```python
from build123d import *

# Parameters (mm, degrees)
F1_W     = 5.5
F1_H     = 15
F1_R     = 1.45
F2_DEPTH = 4
F3_DEPTH = 14
F4_R     = 2.5
F5_R     = 5
F6_W     = 42.5
F6_H     = 2
F7_DEPTH = 4
F8_SIZE2 = 4
F8_SIZE  = 20
F9_R     = 1


with BuildPart() as f2:
    # F1 (on Top) → F2 (new body)
    with BuildSketch(Plane.XY):
        with BuildLine():
            ThreePointArc((-44, 27), (-42.232233047, 26.267766953), (-41.5, 24.5))
            ThreePointArc((-41.5, 24.5), (-44, 22), (-46.5, 24.5))
            Line((-46.5, 24.5), (-46.5, -24.5))
            ThreePointArc((-46.5, -24.5), (-44, -22), (-41.5, -24.5))
            ThreePointArc((-41.5, -24.5), (-42.232233047, -26.267766953), (-44, -27))
            Line((-44, -27), (14, -27))
            Line((14, -27), (16.5, -27))
            Line((16.5, -27), (57.5, -27))
            Line((57.5, -27), (57.5, 27))
            Line((57.5, 27), (16.5, 27))
            Line((16.5, 27), (14, 27))
            Line((14, 27), (-44, 27))
        make_face()
        with BuildLine():
            ThreePointArc((16.5, -24.5), (15.767766953, -26.267766953), (14, -27))
            ThreePointArc((14, -27), (12.232233047, -22.732233047), (16.5, -24.5))
        make_face(mode=Mode.SUBTRACT)
        with Locations((47.5, -12)):
            Rectangle(F1_W, F1_H, mode=Mode.SUBTRACT)
        Polygon((11.5, -19.400605268), (11.5, -22), (8.368910891, -22), (-38.368910891, -22), (-41.5, -22), (-41.5, -19.400605268), (-41.5, 19.400605268), (-41.5, 22), (-38.368910891, 22), (8.368910891, 22), (11.5, 22), (11.5, 19.400605268), align=None, mode=Mode.SUBTRACT)
        with Locations((47.5, 12)):
            Rectangle(F1_W, F1_H, mode=Mode.SUBTRACT)
        with BuildLine():
            ThreePointArc((16.5, 24.5), (12.232233047, 22.732233047), (14, 27))
            ThreePointArc((14, 27), (15.767766953, 26.267766953), (16.5, 24.5))
        make_face(mode=Mode.SUBTRACT)
        Polygon((-41.5, 19.400605268), (-18.131089109, 0), (-15, 2.599394732), (-38.368910891, 22), (-41.5, 22), align=None)
        Polygon((-11.868910891, 0), (11.5, 19.400605268), (11.5, 22), (8.368910891, 22), (-15, 2.599394732), align=None)
        Polygon((8.368910891, -22), (11.5, -22), (11.5, -19.400605268), (-11.868910891, 0), (-15, -2.599394732), align=None)
        Polygon((-41.5, -22), (-38.368910891, -22), (-15, -2.599394732), (-18.131089109, 0), (-41.5, -19.400605268), align=None)
        with BuildLine():
            ThreePointArc((16.5, 24.5), (15.767766953, 26.267766953), (14, 27))
            ThreePointArc((14, 27), (12.232233047, 22.732233047), (16.5, 24.5))
        make_face()
        with Locations((14, 24.5)):
            Circle(F1_R, mode=Mode.SUBTRACT)
        with BuildLine():
            ThreePointArc((16.5, -24.5), (12.232233047, -22.732233047), (14, -27))
            ThreePointArc((14, -27), (15.767766953, -26.267766953), (16.5, -24.5))
        make_face()
        with Locations((14, -24.5)):
            Circle(F1_R, mode=Mode.SUBTRACT)
        with BuildLine():
            ThreePointArc((-46.5, 24.5), (-44, 22), (-41.5, 24.5))
            ThreePointArc((-41.5, 24.5), (-42.232233047, 26.267766953), (-44, 27))
            ThreePointArc((-44, 27), (-45.767766953, 26.267766953), (-46.5, 24.5))
        make_face()
        with Locations((-44, 24.5)):
            Circle(F1_R, mode=Mode.SUBTRACT)
        with BuildLine():
            ThreePointArc((-41.5, -24.5), (-44, -22), (-46.5, -24.5))
            ThreePointArc((-46.5, -24.5), (-45.767766953, -26.267766953), (-44, -27))
            ThreePointArc((-44, -27), (-42.232233047, -26.267766953), (-41.5, -24.5))
        make_face()
        with Locations((-44, -24.5)):
            Circle(F1_R, mode=Mode.SUBTRACT)
        Polygon((-18.131089109, 0), (-15, -2.599394732), (-11.868910891, 0), (-15, 2.599394732), align=None)
    extrude(amount=F2_DEPTH)

    # F1 (on Top) → F3 (join)
    with BuildSketch(Plane.XY):
        with BuildLine():
            ThreePointArc((-46.5, 24.5), (-44, 22), (-41.5, 24.5))
            ThreePointArc((-41.5, 24.5), (-42.232233047, 26.267766953), (-44, 27))
            ThreePointArc((-44, 27), (-45.767766953, 26.267766953), (-46.5, 24.5))
        make_face()
        with Locations((-44, 24.5)):
            Circle(F1_R, mode=Mode.SUBTRACT)
        with BuildLine():
            ThreePointArc((16.5, 24.5), (15.767766953, 26.267766953), (14, 27))
            ThreePointArc((14, 27), (12.232233047, 22.732233047), (16.5, 24.5))
        make_face()
        with Locations((14, 24.5)):
            Circle(F1_R, mode=Mode.SUBTRACT)
        with BuildLine():
            ThreePointArc((16.5, -24.5), (12.232233047, -22.732233047), (14, -27))
            ThreePointArc((14, -27), (15.767766953, -26.267766953), (16.5, -24.5))
        make_face()
        with Locations((14, -24.5)):
            Circle(F1_R, mode=Mode.SUBTRACT)
        with BuildLine():
            ThreePointArc((-41.5, -24.5), (-44, -22), (-46.5, -24.5))
            ThreePointArc((-46.5, -24.5), (-45.767766953, -26.267766953), (-44, -27))
            ThreePointArc((-44, -27), (-42.232233047, -26.267766953), (-41.5, -24.5))
        make_face()
        with Locations((-44, -24.5)):
            Circle(F1_R, mode=Mode.SUBTRACT)
    extrude(amount=F3_DEPTH)

    # F4
    f4_edges = [f2.edges().sort_by_distance(p)[0] for p in [
        (44.75, 19.5, 2),
        (50.25, 19.5, 2),
        (50.25, 4.5, 2),
        (44.75, 4.5, 2),
        (44.75, -19.5, 2),
        (50.25, -19.5, 2),
        (50.25, -4.5, 2),
        (44.75, -4.5, 2),
    ]]
    fillet(f4_edges, radius=F4_R)

    # F5
    f5_edges = [f2.edges().sort_by_distance(p)[0] for p in [
        (57.5, -27, 2),
        (57.5, 27, 2),
    ]]
    fillet(f5_edges, radius=F5_R)

    # F6 (on face) → F7 (join)
    with BuildSketch(Plane.XY.offset(4)):
        with BuildLine():
            ThreePointArc((15, 22.2087121525), (14, 22), (13, 22.2087121525))
            Line((13, 22.2087121525), (13, -22.2087121525))
            ThreePointArc((13, -22.2087121525), (14, -22), (15, -22.2087121525))
            Line((15, -22.2087121525), (15, -1))
            Line((15, -1), (15, 1))
            Line((15, 1), (15, 22.2087121525))
        make_face()
        with Locations((36.25, 0)):
            Rectangle(F6_W, F6_H)
    extrude(amount=F7_DEPTH)

    # F8
    f8_edges = [f2.edges().sort_by_distance(p)[0] for p in [
        (57.5, 0, 8),
    ]]
    f8_side = f2.faces().sort_by_distance((24.914828, 0, 8))[0]
    chamfer(f8_edges, length=F8_SIZE, length2=F8_SIZE2, reference=f8_side)

    # F9
    f9_edges = [f2.edges().sort_by_distance(p)[0] for p in [
        (-41.5, 19.400605, 2),
        (-38.368911, 22, 2),
        (8.368911, 22, 2),
        (11.5, 19.400605, 2),
        (11.5, -19.400605, 2),
        (8.368911, -22, 2),
        (-38.368911, -22, 2),
        (-41.5, -19.400605, 2),
        (-18.131089, 0, 2),
        (-15, -2.599395, 2),
        (-11.868911, 0, 2),
        (-15, 2.599395, 2),
    ]]
    fillet(f9_edges, radius=F9_R)


solid = f2.part
```
For this review, take the finished solid that the model builds, in its own axes (mm). A direction names the side the tool comes from. Round coordinates to 2 decimals unless told otherwise and drop trailing zeros. Loops run counter-clockwise (first coordinate to the right, second up) from the corner with the lowest first, then second, coordinate; pieces in that order, holes last.
(1) Tool access review of faces 1 (the flat face through (15, -12, 6)), 2 (the flat face through (11.5, 0, 2)), 3 (the flat face through (-17, 0, 4)): name each direction out of +Z, -Z, +X, -X, +Y, -Y from which nothing blocks a thin tool from reaching the whole face with its end or side.
Returned:
face 1: +Z, +X
face 2: +Z, -Z
face 3: +Z
(2) Mouldability with a two-part tool opening along Y and no side actions: class faces 4 (the flat face through (47.64, -0.01, 5.97)), 5 (the cylindrical face through (56.07, 25.5, 2.03)), 6 (the flat face through (-15, 22, 2)) as released by +Y, released by -Y, zero draft, split by the parting line, or undercut.
Returned:
face 4: zero draft
face 5: released by +Y
face 6: undercut
(3) Clearance check with flat-ended pins moving along their axes: P1, Ø10, axis at x = 7, y = -1, coming from the -Z side; P2, Ø4.5, axis at y = -11.5, z = 6.5, coming from the +X side; P3, Ø2.5, axis at x = -44, y = -24.5, coming from the +Z side; P4, Ø13, axis at x = 44.5, y = 15, coming from the +Z side. State where each tip first meets the part, or that it passes through.
Returned:
P1: stops at z = 0
P2: stops at x = 15
P3: passes through
P4: stops at z = 4
(4) We need section C-C (x = 4.5). Give the boundary of the cut face in (y, z), plus the area to 3 significant figures.
Returned:
outline: (-27, 0) - (-22, 0) - (-22, 4) - (-27, 4) - close; (-18.79, 0) - (-13.59, 0) - (-13.59, 4) - (-18.79, 4) - close; (13.59, 0) - (18.79, 0) - (18.79, 4) - (13.59, 4) - close; (22, 0) - (27, 0) - (27, 4) - (22, 4) - close
area: 81.6 mm2
(5) We need section B-B (z = 5.75). Give the boundary of the cut face in (x, y), plus the area to 3 significant figures.
Returned:
outline: circle Ø5 at (-44, -24.5); circle Ø5 at (-44, 24.5); (13, -22.21) arc R2.5 ccw (long way) to (15, -22.21) - (15, -1) - (48.75, -1) - (48.75, 1) - (15, 1) - (15, 22.21) arc R2.5 ccw (long way) to (13, 22.21) - close; hole circle Ø2.9 at (-44, -24.5); hole circle Ø2.9 at (-44, 24.5); hole circle Ø2.9 at (14, -24.5); hole circle Ø2.9 at (14, 24.5)
area: 208 mm2
(6) We need section D-D (y = 9). Give the boundary of the cut face in (x, z), plus the area to 3 significant figures.
Returned:
outline: (-46.5, 0) - (-41.5, 0) - (-41.5, 4) - (-46.5, 4) - close; (-28.97, 0) - (-22.71, 0) - (-22.71, 4) - (-28.97, 4) - close; (-7.29, 0) - (-1.03, 0) - (-1.03, 4) - (-7.29, 4) - close; (11.5, 0) - (44.75, 0) - (44.75, 4) - (15, 4) - (15, 8) - (13, 8) - (13, 4) - (11.5, 4) - close; (50.25, 0) - (57.5, 0) - (57.5, 4) - (50.25, 4) - close
area: 240 mm2
(7) We need section A-A (z = 11.5). Give the boundary of the cut face in (x, y).
Returned:
outline: circle Ø5 at (-44, -24.5); circle Ø5 at (-44, 24.5); circle Ø5 at (14, -24.5); circle Ø5 at (14, 24.5); hole circle Ø2.9 at (-44, -24.5); hole circle Ø2.9 at (-44, 24.5); hole circle Ø2.9 at (14, -24.5); hole circle Ø2.9 at (14, 24.5)
(8) Wall thickness on line 1 along Y through (x, z) = (14, 11.25); line 2 along Y through (x, z) = (14, 6); line 3 along X through (y, z) = (-6, 1.25): over which ranges is each line inside the solid? List them lowest first.
Returned:
line 1: y = -27 to -25.95, -23.05 to -22, 22 to 23.05, 25.95 to 27
line 2: y = -27 to -25.95, -23.05 to 23.05, 25.95 to 27
line 3: x = -46.5 to -41.5, -25.36 to -19.1, -10.9 to -4.64, 11.5 to 44.96, 50.04 to 57.5
